The model under review builds one solid part; all positions refer to its coordinate system, in mm. A direction names the side the tool comes from. Give positions to 0.01 mm unless a question says otherwise; leave off trailing zeros. Order: outer loops, then holes, each group sorted by start corner. A loop starts at its lowest first (then second) coordinate and runs counter-clockwise, first axis right, second up. Notation, with made-up numbers: (69.25, 1.5) -> (91.25, 1.5) arc R22 ccw to (91.25, 40.5) -> close; hole circle Ø4 at (72, -10). An arc over 180 degrees is marked (long way). Use one line per item in the form item = value.
```python
from build123d import *

# Parameters (mm, degrees)
F1_DEPTH = 2
F3_DEPTH = 25.4
F4_R     = 2.9673782323
F5_DEPTH = 25.4


with BuildPart() as f1:
    # F0 (on Top) → F1 (new body)
    with BuildSketch(Plane.XY):
        with BuildLine():
            Line((36.5334041417, 20.6077042967), (34.7164385021, 5.6545715779))
            Line((34.7164385021, 5.6545715779), (43.504524976, 8.7329633534))
            Line((43.504524976, 8.7329633534), (53.3858016133, 22.3565343767))
            Line((53.3858016133, 22.3565343767), (56.9245554507, 23.5919579864))
            Line((56.9245554507, 23.5919579864), (66.0541206598, 3.5111056641))
            Line((66.0541206598, 3.5111056641), (65.5934512615, 0.3702012473))
            Line((65.5934512615, 0.3702012473), (88.8780280948, 8.5993725806))
            Line((88.8780280948, 8.5993725806), (77.8220444918, 9.6044624224))
            Line((77.8220444918, 9.6044624224), (79.9770836988, 33.3098837159))
            add(Edge.make_bspline(
                [(100.9928658605, 43.4244535863), (95.8205314108, 40.4245140318), (87.218727926, 35.4354920021), (82.0412871818, 33.9157803728), (79.9770836988, 33.3098837159)],
                knots=[0, 0, 0, 0, 0.6013081395, 1, 1, 1, 1], degree=3))
            Line((100.9928658605, 43.4244535863), (122.4057301879, 56.8480975926))
            Line((122.4057301879, 56.8480975926), (100.9928658605, 54.5836277306))
            add(Edge.make_bspline(
                [(74.1065740585, 48.7466789782), (77.7375523931, 49.9883488185), (85.5402467252, 52.6566022015), (95.6093908771, 53.9122791626), (100.9928658605, 54.5836277306)],
                knots=[0, 0, 0, 0, 0.4653492986, 1, 1, 1, 1], degree=3))
            Line((74.1065740585, 48.7466789782), (56.1992712319, 65.4858723283))
            Line((56.1992712319, 65.4858723283), (64.1599148512, 73.2015818357))
            Line((64.1599148512, 73.2015818357), (40.3392016888, 64.9551600218))
            Line((40.3392016888, 64.9551600218), (43.0131666362, 62.9139691591))
            Line((43.0131666362, 62.9139691591), (49.7575812042, 42.1915054321))
            Line((49.7575812042, 42.1915054321), (46.0408888757, 40.785189718))
            Line((46.0408888757, 40.785189718), (28.6829099059, 45.0443252921))
            Line((28.6829099059, 45.0443252921), (20.3454550356, 41.9102460146))
            Line((20.3454550356, 41.9102460146), (32.1155525744, 31.5474160016))
            Line((32.1155525744, 31.5474160016), (34.8427295685, 31.390786171))
            Line((34.8427295685, 31.390786171), (26.7557948828, 23.5558375716))
            Line((26.7557948828, 23.5558375716), (38.4109728038, 22.2089737654))
            Line((38.4109728038, 22.2089737654), (36.5334041417, 20.6077042967))
        make_face()
    extrude(amount=F1_DEPTH)

    # F2 (on face) → F3 (cut)
    with BuildSketch(Plane.XY.offset(2)):
        with BuildLine():
            Line((42.2181976585, 19.8732110921), (36.8692806095, 17.4346802651))
            Line((36.8692806095, 17.4346802651), (36.4842974601, 15.086657103))
            Line((36.4842974601, 15.086657103), (46.7783554459, 19.8987160716))
            add(Edge.make_bspline(
                [(46.7783554459, 19.8987160716), (46.8745176, 19.9704084061), (47.0739666013, 20.1191047892), (47.2980762453, 20.485200609), (47.3842570525, 20.8264985477), (47.4302483861, 21.0086359383)],
                knots=[0, 0, 0, 0, 0.3027331314, 0.6278958833, 1, 1, 1, 1], degree=3))
            Line((47.4302483861, 21.0086359383), (47.7455708418, 31.8560887995))
            Line((47.7455708418, 31.8560887995), (81.0400521274, 47.3815603972))
            Line((81.0400521274, 47.3815603972), (62.989893266, 40.6838828661))
            add(Edge.make_bspline(
                [(62.989893266, 40.6838828661), (62.8558315332, 40.6463925764), (62.5252333481, 40.5539409762), (61.561398363, 40.2753929938), (60.1603447931, 40.0500849593), (58.6709939197, 39.9709989719), (57.7632965831, 39.984203494), (57.3223569205, 39.9906179643)],
                knots=[0, 0, 0, 0, 0.128570723, 0.3170572751, 0.5463912938, 0.7796467371, 1, 1, 1, 1], degree=3))
            Line((57.3223569205, 39.9906179643), (52.6017494717, 40.801062884))
            Line((52.6017494717, 40.801062884), (57.934057, 37.1581308102))
            Line((57.934057, 37.1581308102), (42.6651981272, 30.0381449865))
            Line((42.6651981272, 30.0381449865), (42.2181976585, 19.8732110921))
        make_face()
        Polygon((49.5022008402, 30.2405287443), (49.0949496514, 20.9795062106), (59.8999263935, 26.0145180069), (59.9547064443, 27.8990143615), (54.1489528303, 25.2522151997), (54.2186230073, 26.8365373498), (58.1639420177, 28.6762698182), (58.2499672688, 30.6325115923), (54.2469362683, 28.8075600354), (54.2916153656, 30.3445720468), (58.3938732965, 32.2574863357), (58.4538725188, 34.3215281581), align=None)
        Polygon((59.5222907582, 34.9345568584), (59.428932466, 32.8115593767), (59.4646008131, 32.7350683593), (61.9832756911, 33.9087458252), (61.6749329049, 26.8969320603), (66.5988146686, 29.1416925155), (66.910579019, 36.231313745), (69.3646524393, 37.3756669746), (69.4611082747, 39.5691035793), align=None)
        with BuildLine():
            Line((68.6329693369, 31.9457548078), (68.5782904095, 30.0647372126))
            Line((68.5782904095, 30.0647372126), (78.7814682825, 34.8225571923))
            Line((78.7814682825, 34.8225571923), (78.8403507658, 38.8965850372))
            add(Edge.make_bspline(
                [(78.2723558252, 39.7925434403), (78.3906581343, 39.7604877829), (78.6166051238, 39.6992643009), (78.8326978206, 39.4449395511), (78.8350317991, 39.281221064), (78.8383302277, 39.0426983364), (78.8403507658, 38.8965850372)],
                knots=[0, 0, 0, 0, 0.2775927016, 0.5301776076, 0.7121980765, 1, 1, 1, 1], degree=3))
            Line((78.2723558252, 39.7925434403), (73.6286103285, 39.3689603356))
            Line((73.6286103285, 39.3689603356), (78.8465645596, 41.8021323534))
            Line((78.8465645596, 41.8021323534), (79.0354909806, 44.0337115572))
            Line((79.0354909806, 44.0337115572), (70.9420511465, 40.2596785817))
            add(Edge.make_bspline(
                [(70.3706405965, 39.3610387878), (70.3940565505, 39.4260226012), (70.4447676448, 39.5667557219), (70.5089015879, 39.8524246499), (70.812566625, 40.1149514275), (70.9043252634, 40.2175116908), (70.9420511465, 40.2596785817)],
                knots=[0, 0, 0, 0, 0.2238252163, 0.4847302664, 0.788150674, 1, 1, 1, 1], degree=3))
            Line((70.3706405965, 39.3610387878), (70.2906058242, 36.2328217133))
            add(Edge.make_bspline(
                [(70.9504246956, 34.8178355773), (70.8567559171, 34.8408667038), (70.6527174927, 34.8910353388), (70.2713296013, 35.1507757935), (70.2107102416, 35.6389400995), (70.2627540341, 36.0257931705), (70.2906058242, 36.2328217133)],
                knots=[0, 0, 0, 0, 0.2072963417, 0.4515530113, 0.7064927503, 1, 1, 1, 1], degree=3))
            Line((70.9504246956, 34.8178355773), (75.0539136601, 35.1847569247))
            Line((75.0539136601, 35.1847569247), (68.6329693369, 31.9457548078))
        make_face()
    extrude(amount=-F3_DEPTH, mode=Mode.SUBTRACT)

    # F4 (on face) → F5 (cut)
    with BuildSketch(Plane.XY.offset(2)):
        with Locations((49.6815554798, 63.3011460304)):
            Circle(F4_R)
    extrude(amount=-F5_DEPTH, mode=Mode.SUBTRACT)


solid = f1.part
```
1. Add section C-C on z = 1.5. Count the separate pieces of the cut face and the enclosed holes in it, then the cut area to 3 significant figures.
Values:
separate_pieces = 1
enclosed_holes = 5
area = 2,270 mm^2
2. Tool access review of faces 5 (the face through (26.15, 36.8, 0.99)), 6 (the face through (56.314, 31.288, 1.014)): name each direction out of +Z, -Z, +X, -X, +Y, -Y from which nothing blocks a thin tool from reaching the whole face with its end or side.
Values:
face_5 = +Z, -Z, -X
face_6 = +Z, -Z
3. For L1, parallel to Y at x = 53.5, z = 0.5; L2, parallel to X at y = 29.5, z = 0.6; L3, parallel to X at y = 18, z = 0.4, list the stretches that pass through material, from the lowest coordinate up.
Values:
L1 = 22.4 to 23.03, 32.06 to 34.54, 35.09 to 40.19, 40.65 to 69.51
L2 = 32.89 to 42.64, 47.68 to 49.47, 54.27 to 55.77, 58.2 to 61.79, 66.61 to 79.63
L3 = 36.22 to 38.11, 42.72 to 50.23, 59.47 to 78.59
4. Add section A-A on x = 45. Give the boundary of the cut face in (y, z).
Values:
outline = (10.79, 0) -> (19.07, 0) -> (19.07, 2) -> (10.79, 2) -> close; (31.13, 0) -> (41.04, 0) -> (41.04, 2) -> (31.13, 2) -> close; (56.81, 0) -> (66.57, 0) -> (66.57, 2) -> (56.81, 2) -> close
5. Add section B-B on y = 59. Give the boundary of the cut face in (x, z).
Values:
outline = (44.29, 0) -> (63.14, 0) -> (63.14, 2) -> (44.29, 2) -> close
6. Add section D-D on x = 107.5. Give the boundary of the cut face in (y, z).
Values:
outline = (47.5, 0) -> (55.27, 0) -> (55.27, 2) -> (47.5, 2) -> close
7. The part is to be moulded in two halves that separate along Y. For faces 1 (the face through (78.884, 21.291, 0.986)), 2 (the face through (48.376, 15.449, 0.986)), 3 (the face through (35.64, 13.24, 0.99)), 4 (the face through (67, 40, 0)), say which applies: +Y half, -Y half, draft (parallel to the pull), parting line (faces both ways), or undercut.
Values:
face_1 = undercut
face_2 = -Y half
face_3 = undercut
face_4 = draft
8. For pin 1 Ø6 at (x, y) = (85.5, 29) entering from -Z, flat-tipped, find the tip position at first contact; note if it passes through.
Values:
pin_1 = through
